from build123d import *

# Parameters (mm, degrees)
F1_DEPTH  = 4
F2_R      = 8.05
F3_DEPTH  = 4.001
F4_W      = 10
F4_H      = 45
F5_DEPTH  = 25
F6_R      = 1.75
F7_DEPTH  = 29.001
F8_R      = 1.75
F9_DEPTH  = 29.001
F10_R     = 3
F11_R     = 4
F12_R     = 3
F13_DEPTH = 4.001


with BuildPart() as f1:
    # F0 (on Front) → F1 (new body)
    with BuildSketch(Plane.XZ):
        with BuildLine():
            Line((45, 22.5), (-45, 22.5))
            ThreePointArc((-45, 22.5), (-67.5, 0), (-45, -22.5))
            Line((-45, -22.5), (45, -22.5))
            Line((45, -22.5), (45, 22.5))
        make_face()
    extrude(amount=F1_DEPTH)

    # F2 (on face) → F3 (cut, through all)
    with BuildSketch(Plane.XZ.offset(4)):
        with Locations((-45, 0)):
            Circle(F2_R)
    extrude(amount=-F3_DEPTH, mode=Mode.SUBTRACT)

    # F4 (on face) → F5 (join)
    with BuildSketch(Plane.XZ.offset(4)):
        Polygon((-0.3, 6.9010445144), (-22, 12.5778352683), (-22, 0), (-22, -12.5778352683), (-0.3, -6.9010445144), (-0.3, 0), align=None)
        with Locations((40, 0)):
            Rectangle(F4_W, F4_H)
    extrude(amount=F5_DEPTH)

    # F6 (on face) → F7 (cut, through all)
    with BuildSketch(Plane.XZ.offset(29)):
        with Locations((-16, 0)):
            Circle(F6_R)
        with Locations((-6.3, 0)):
            Circle(F6_R)
    extrude(amount=-F7_DEPTH, mode=Mode.SUBTRACT)

    # F8 (on face) → F9 (cut, through all)
    with BuildSketch(Plane.XZ.offset(29)):
        with Locations((40, 16.5)):
            Circle(F8_R)
        with Locations((40, -16.5)):
            Circle(F8_R)
    extrude(amount=-F9_DEPTH, mode=Mode.SUBTRACT)

    # F10
    f10_edges = [f1.edges().sort_by_distance(p)[0] for p in [
        (-0.3, -16.5, 6.901045),
        (-22, -16.5, 12.577835),
        (-22, -16.5, -12.577835),
        (-0.3, -16.5, -6.901045),
    ]]
    fillet(f10_edges, radius=F10_R)

    # F11
    f11_edges = [f1.edges().sort_by_distance(p)[0] for p in [
        (45, -14.5, 22.5),
        (45, -14.5, -22.5),
        (35, -16.5, 22.5),
        (35, -16.5, -22.5),
    ]]
    fillet(f11_edges, radius=F11_R)

    # F12 (on face) → F13 (cut, through all)
    with BuildSketch(Plane.XZ.offset(4)):
        with Locations((-3.8, 15.5)):
            Circle(F12_R)
        with Locations((-3.8, -15.5)):
            Circle(F12_R)
        with Locations((27.2, -15.5)):
            Circle(F12_R)
        with Locations((27.2, 15.5)):
            Circle(F12_R)
    extrude(amount=-F13_DEPTH, mode=Mode.SUBTRACT)


solid = f1.part
For this review, take the finished solid that the model builds, in its own axes (mm). A direction names the side the tool comes from. Round coordinates to 2 decimals unless told otherwise and drop trailing zeros. Order: outer loops, then holes, each group sorted by start corner. A loop starts at its lowest first (then second) coordinate and runs counter-clockwise, first axis right, second up. Notation, with made-up numbers: (6.25, -28.75) -> (62.25, -28.75) arc R6 ccw to (62.25, -23.75) -> close; hole circle Ø6 at (6.5, -32.75). An arc over 180 degrees is marked (long way). Write item = value, one per line. Start each with the question number.
1) Tool access review of faces 1 (the face through (-0.3, -16, 0)), 2 (the face through (-10.5, -16.32, -9.57)), 3 (the face through (36.141, -16.675, 21.297)), 4 (the face through (36.141, -16.675, -21.297)): name each direction out of +Z, -Z, +X, -X, +Y, -Y from which nothing blocks a thin tool from reaching the whole face with its end or side.
2) The part is to be moulded in two halves that separate along X. For faces 5 (the face through (43.797, -14.297, 21.359)), 6 (the face through (4, -3, 22.5)), 7 (the face through (-10.28, -16.32, 9.51)), say which applies: +X half, -X half, draft (parallel to the pull), parting line (faces both ways), or undercut.
3) Take a section at C-C on x = -16. State the section outline as (y, z) points.
4) Insertion check: pin 1 (10 mm diameter, centred on x = -38.5, z = -17.5, fed in from -Y); pin 2 (5.5 mm diameter, centred on x = -3.8, z = 15.5, fed in from -Y); pin 3 (8 mm diameter, centred on y = -16.5, z = 6.5, fed in from -X); pin 4 (5 mm diameter, centred on y = -23.5, z = 13.5, fed in from -X). Each pin has a flat end and moves straight along its axis. Give the tip position at first contact, or say it passes through.
5) To check wall thickness, follow line 1 (Z direction, x = 27.2, y = -1.3); line 2 (Z direction, x = 40, y = -7.75); line 3 (X direction, y = -18.25, z = 4.5). State the ranges of each line that lie inside material, in increasing order. Write a range as from..to.
6) Take a section at D-D on x = 27.2. State the section outline as (y, z) points.
7) Take a section at A-A on y = -19.25. State the section outline as (x, z) points, plus the area to 3 significant figures.
8) Take a section at B-B on x = 40. State the section outline as (y, z) points, plus the area to 3 significant figures.
Verdict:
q1.face_1 = +Z, -Z, -Y
q1.face_2 = -Z, -Y
q1.face_3 = +Z, -X, -Y
q1.face_4 = -Z, -X, -Y
q2.face_5 = +X half
q2.face_6 = draft
q2.face_7 = undercut
q3.outline = (-29, -11.01) -> (-4, -11.01) -> (-4, -22.5) -> (0, -22.5) -> (0, -1.75) -> (-29, -1.75) -> close; (-29, 1.75) -> (0, 1.75) -> (0, 22.5) -> (-4, 22.5) -> (-4, 11.01) -> (-29, 11.01) -> close
q4.pin_1 = -4
q4.pin_2 = through
q4.pin_3 = -22
q4.pin_4 = -20.92
q5.line_1 = -22.5..-18.5, -12.5..12.5, 18.5..22.5
q5.line_2 = -22.5..-18.25, -14.75..14.75, 18.25..22.5
q5.line_3 = -22..-0.3, 35..45
q6.outline = (-4, -22.5) -> (0, -22.5) -> (0, -18.5) -> (-4, -18.5) -> close; (-4, -12.5) -> (0, -12.5) -> (0, 12.5) -> (-4, 12.5) -> close; (-4, 18.5) -> (0, 18.5) -> (0, 22.5) -> (-4, 22.5) -> close
q7.outline = (-22, -8.69) arc R3 ccw to (-18.24, -11.59) -> (-2.54, -7.49) arc R3 ccw to (-0.3, -4.58) -> (-0.3, 4.58) arc R3 ccw to (-2.54, 7.49) -> (-18.24, 11.59) arc R3 ccw to (-22, 8.69) -> close; (35, -18.5) arc R4 ccw to (39, -22.5) -> (41, -22.5) arc R4 ccw to (45, -18.5) -> (45, 18.5) arc R4 ccw to (41, 22.5) -> (39, 22.5) arc R4 ccw to (35, 18.5) -> close; hole circle Ø3.5 at (-16, 0); hole circle Ø3.5 at (-6.3, 0); hole circle Ø3.5 at (40, -16.5); hole circle Ø3.5 at (40, 16.5)
q7.area = 812 mm2
q8.outline = (-29, -22.5) -> (0, -22.5) -> (0, -18.25) -> (-29, -18.25) -> close; (-29, -14.75) -> (0, -14.75) -> (0, 14.75) -> (-29, 14.75) -> close; (-29, 18.25) -> (0, 18.25) -> (0, 22.5) -> (-29, 22.5) -> close
q8.area = 1,100 mm2
